Design review of the part built by this model. Coordinates are the model's own, in mm. A direction names the side the tool comes from. Coordinates: 2 decimals unless noted, no trailing zeros. Write each loop counter-clockwise with the first axis right and the second up, starting at its lowest first coordinate (ties: lowest second). Pieces come first, ordered by that corner, then holes.
Q1. Take a section at A-A (z = 0). Give the boundary of the cut face in (x, y).
Q2. Take a section at D-D (x = 3.25). Give the boundary of the cut face in (y, z).
Q3. Machinability: for faces 1 (the flat face through (4.85, -1, -1)), 2 (the cylindrical face through (17.542, 0.323, -0.506)), 3 (the cylindrical face through (3.33, -1.27, 0.97)), which of the approach directions +Z, -Z, +X, -X, +Y, -Y give a long, thin tool a straight path to every point of the face, cutting with its end or side? Answer none if there is none.
Q4. Take a section at C-C (x = 10.25). Give the boundary of the cut face in (y, z), and give its area (3 significant figures).
Q5. For probe 1 along X at (y, z) = (1, 0.55); probe 2 along X at (y, z) = (0.3, -0.85); probe 3 along Z at (x, y) = (4.5, 1.3), list the stretches that pass through material, from the lowest coordinate up.
Q6. Mouldability with a two-part tool opening along X and no side actions: class faces 4 (the cylindrical face through (18.396, -0.217, 0.976)), 5 (the flat face through (19.1, 0, 0)), 6 (the flat face through (1.85, -1, -1)) as pulls with the +X half, pulls with the -X half, needs draft (parallel to the pull), parting line crosses it, or undercut.
Q7. Insertion check: pin 1 (1.5 mm diameter, centred on x = 16, z = -1, fed in from +Y). The pin has a flat end and moves straight along its axis. Give the tip position at first contact, or say it passes through.
Autodesk Inventor part; units mm, degrees
ref_plane "YZ Plane" through (0, 0, 0) normal (1, 0, 0) x (0, 1, 0)
ref_plane "XZ Plane" through (0, 0, 0) normal (0, 1, 0) x (-1, 0, 0)
ref_plane "XY Plane" through (0, 0, 0) normal (0, 0, 1) x (1, 0, 0)
sketch "Sketch1" plane through (0, 0, 0) normal (0, 0, 1) x (1, 0, 0)
  line L0 (0, 0) -> (1.1, 0)
  line L1 (1.1, 0) -> (1.1, 1.6)
  line L2 (1.1, 1.6) -> (0, 1.6)
  line L3 (0, 1.6) -> (0, 0)
  line L4 (1.1, 0) -> (1.85, 0)
  line L5 (1.85, 0) -> (1.85, 1)
  line L6 (1.85, 1) -> (1.1, 1)
  line L7 (1.1, 1) -> (1.1, 0)
  line L8 (1.85, 0) -> (4.85, 0)
  line L9 (4.85, 0) -> (4.85, 1.6)
  line L10 (4.85, 1.6) -> (1.85, 1.6)
  line L11 (1.85, 1.6) -> (1.85, 0)
  line L12 (4.85, 0) -> (17, 0)
  line L13 (17, 0) -> (17, 1)
  line L14 (17, 1) -> (4.85, 1)
  line L15 (4.85, 1) -> (4.85, 0)
  line L16 (17, 0) -> (18.1, 0)
  line L17 (18.1, 0) -> (18.1, 0.6)
  line L18 (18.1, 0.6) -> (17, 0.6)
  line L19 (17, 0.6) -> (17, 0)
  line L20 (18.1, 0) -> (19.1, 0)
  line L21 (19.1, 0) -> (19.1, 1)
  line L22 (19.1, 1) -> (18.1, 1)
  line L23 (18.1, 1) -> (18.1, 0)
  dimension "d0" = 1.1
  dimension "d1" = 1.85
  dimension "d2" = 4.85
  dimension "d3" = 19.1
  dimension "d4" = 18.1
  dimension "d5" = 17
  dimension "d6" = 2
  dimension "d7" = 1.2
  dimension "d8" = 3.2
  dimension "d9" = 2
revolve "Revolution1" add sketch "Sketch1" angle 360 about axis through (0, 0, 0) along (1, 0, 0)
chamfer "Chamfer1" distance 0.4 angle 45 1 edges at (19.1, -1, 0)
properties part number "403-13" material "Steel"
Response:
1. outline: (0, -1.6) - (1.1, -1.6) - (1.1, -1) - (1.85, -1) - (1.85, -1.6) - (4.85, -1.6) - (4.85, -1) - (17, -1) - (17, -0.6) - (18.1, -0.6) - (18.1, -1) - (18.7, -1) - (19.1, -0.6) - (19.1, 0.6) - (18.7, 1) - (18.1, 1) - (18.1, 0.6) - (17, 0.6) - (17, 1) - (4.85, 1) - (4.85, 1.6) - (1.85, 1.6) - (1.85, 1) - (1.1, 1) - (1.1, 1.6) - (0, 1.6) - close
2. outline: circle Ø3.2 at (0, 0)
3. face 1: +X
3. face 2: none
3. face 3: +X, -X
4. outline: circle Ø2 at (0, 0)
4. area: 3.14 mm2
5. probe 1: x = 0 to 1.1, 1.85 to 4.85
5. probe 2: x = 0 to 17, 18.1 to 18.8
5. probe 3: z = -0.93 to 0.93
6. face 4: needs draft
6. face 5: pulls with the +X half
6. face 6: undercut
7. pin 1: stops at y = 0.97
